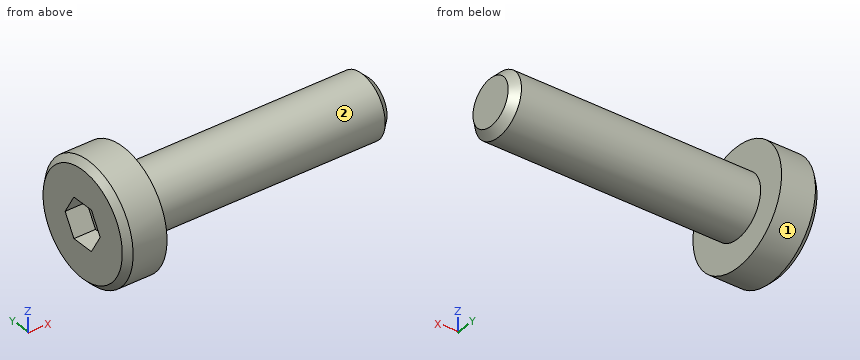
from build123d import *

# Parameters (mm, degrees)
CUT_EXTRUDE1_DEPTH = 0.7


with BuildPart() as part:
    # Sketch1 → Revolve1 (revolve)
    with BuildSketch(Plane.XY):
        Polygon((-1.3, 0), (-1.3, 1.7), (-1.1, 1.9), (0, 1.9), (0, 1), (7.7545, 1), (8, 0.7545), (8, 0), align=None)
    revolve(axis=Axis((8, 0, 0), (-1, 0, 0)))

    # Sketch2 → Cut-Extrude1 (cut)
    with BuildSketch(Plane(origin=(-1.3, 0, 0), x_dir=(0, 0, -1), z_dir=(1, 0, 0))):
        Polygon((-0.65, -0.375277675), (0, -0.75055535), (0.65, -0.375277675), (0.65, 0.375277675), (0, 0.75055535), (-0.65, 0.375277675), align=None)
    extrude(amount=CUT_EXTRUDE1_DEPTH, mode=Mode.SUBTRACT)


solid = part.part
Could you check a few things on this model? Use its own coordinates, in mm. Face numbers are marked on the shaded views. A direction names the side the tool comes from. Give positions to 0.01 mm unless a question says otherwise; leave off trailing zeros. Loops run counter-clockwise (first coordinate to the right, second up) from the corner with the lowest first, then second, coordinate; pieces in that order, holes last. Notation, with made-up numbers: (-6.5, 34) -> (47.5, 34) arc R18 cw to (47.5, 62) -> close; hole circle Ø2 at (60.5, 64.25). An arc over 180 degrees is marked (long way). Answer as CSV lines item,"result". Start each with the question number.
(1) I'm going to push a flat-ended pin straight in: pin 1 Ø1 at (y, z) = (0, 0) entering from -X. Where does the tip first touch, or does it pass through?
(2) I need wall thicknesses on probe 1 along X at (y, z) = (-0.75, 0.85); probe 2 along X at (y, z) = (-0.3, 0.6); probe 3 along Y at (x, z) = (2.75, -0.05). Which ranges of each line are inside material? Lowest first, please.
(3) Which directions (+Z, -Z, +X, -X, +Y, -Y) give clear straight access to the entire face, cutting with the end or side of a thin tool? Please do the marked faces 1 and 2.
(4) If we section it at B-B on x = 4: Write out the boundary of the cut face in (y, z).
(5) If we section it at C-C on x = -0.25: Write out the boundary of the cut face in (y, z), then the cut area to 3 significant figures.
(6) If we section it at A-A on y = 0: Write out the boundary of the cut face in (x, z).
Computed:
1,pin 1,"stops at x = -0.6"
2,probe 1,"x = -1.3 to 0"
2,probe 2,"x = -0.6 to 8"
2,probe 3,"y = -1 to 1"
3,face 1,"+X, -X"
3,face 2,"+X"
4,outline,"circle Ø2 at (0, 0)"
5,outline,"circle Ø3.8 at (0, 0)"
5,area,"11.3 mm2"
6,outline,"(-1.3, -1.7) -> (-1.1, -1.9) -> (0, -1.9) -> (0, -1) -> (7.75, -1) -> (8, -0.75) -> (8, 0.75) -> (7.75, 1) -> (0, 1) -> (0, 1.9) -> (-1.1, 1.9) -> (-1.3, 1.7) -> (-1.3, 0.65) -> (-0.6, 0.65) -> (-0.6, -0.65) -> (-1.3, -0.65) -> close"
